Verification items for the finished model (mm, model axes). Face numbers are marked on the shaded views. A direction names the side the tool comes from. Give positions to 0.01 mm unless a question says otherwise; leave off trailing zeros. Write each loop counter-clockwise with the first axis right and the second up, starting at its lowest first coordinate (ties: lowest second). Pieces come first, ordered by that corner, then holes. Notation, with made-up numbers: (58, 9.25) - (108, 9.25) arc R15 cw to (108, 19.25) - close; hole circle Ø7 at (11, -34). An arc over 180 degrees is marked (long way). Put each result on its own line as item: value.
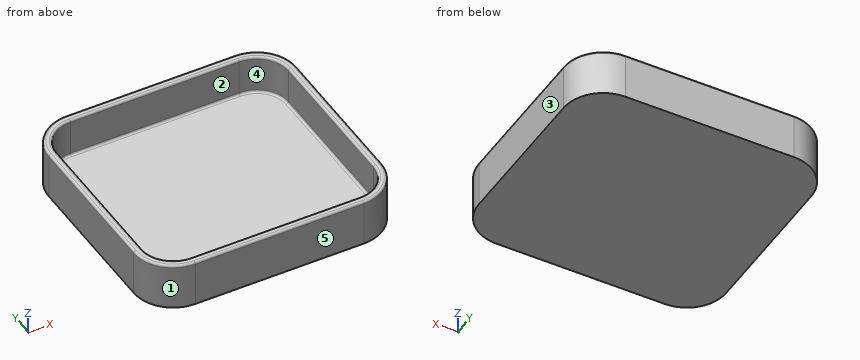
from build123d import *

# Parameters (mm, degrees)
F1_DEPTH = 2.5
F2_DEPTH = 15
F3_R     = 0.75


with BuildPart() as f1:
    # F0 (on Top) → F1 (new body)
    with BuildSketch(Plane.XY):
        with BuildLine():
            Line((26.75, 36.5), (-26.75, 36.5))
            ThreePointArc((-26.75, 36.5), (-35.5888347648, 32.8388347648), (-39.25, 24))
            Line((-39.25, 24), (-39.25, -24))
            ThreePointArc((-39.25, -24), (-35.5888347648, -32.8388347648), (-26.75, -36.5))
            Line((-26.75, -36.5), (26.75, -36.5))
            ThreePointArc((26.75, -36.5), (35.5888347648, -32.8388347648), (39.25, -24))
            Line((39.25, -24), (39.25, 24))
            ThreePointArc((39.25, 24), (35.5888347648, 32.8388347648), (26.75, 36.5))
        make_face()
        with BuildLine():
            ThreePointArc((-36.75, 24), (-33.8210678119, 31.0710678119), (-26.75, 34))
            Line((-26.75, 34), (26.75, 34))
            ThreePointArc((26.75, 34), (33.8210678119, 31.0710678119), (36.75, 24))
            Line((36.75, 24), (36.75, -24))
            ThreePointArc((36.75, -24), (33.8210678119, -31.0710678119), (26.75, -34))
            Line((26.75, -34), (-26.75, -34))
            ThreePointArc((-26.75, -34), (-33.8210678119, -31.0710678119), (-36.75, -24))
            Line((-36.75, -24), (-36.75, 24))
        make_face(mode=Mode.SUBTRACT)
        with BuildLine():
            Line((26.75, 34), (-26.75, 34))
            ThreePointArc((-26.75, 34), (-33.8210678119, 31.0710678119), (-36.75, 24))
            Line((-36.75, 24), (-36.75, -24))
            ThreePointArc((-36.75, -24), (-33.8210678119, -31.0710678119), (-26.75, -34))
            Line((-26.75, -34), (26.75, -34))
            ThreePointArc((26.75, -34), (33.8210678119, -31.0710678119), (36.75, -24))
            Line((36.75, -24), (36.75, 24))
            ThreePointArc((36.75, 24), (33.8210678119, 31.0710678119), (26.75, 34))
        make_face()
    extrude(amount=F1_DEPTH)

    # F0 (on Top) → F2 (join)
    with BuildSketch(Plane.XY):
        with BuildLine():
            Line((26.75, 36.5), (-26.75, 36.5))
            ThreePointArc((-26.75, 36.5), (-35.5888347648, 32.8388347648), (-39.25, 24))
            Line((-39.25, 24), (-39.25, -24))
            ThreePointArc((-39.25, -24), (-35.5888347648, -32.8388347648), (-26.75, -36.5))
            Line((-26.75, -36.5), (26.75, -36.5))
            ThreePointArc((26.75, -36.5), (35.5888347648, -32.8388347648), (39.25, -24))
            Line((39.25, -24), (39.25, 24))
            ThreePointArc((39.25, 24), (35.5888347648, 32.8388347648), (26.75, 36.5))
        make_face()
        with BuildLine():
            ThreePointArc((-36.75, 24), (-33.8210678119, 31.0710678119), (-26.75, 34))
            Line((-26.75, 34), (26.75, 34))
            ThreePointArc((26.75, 34), (33.8210678119, 31.0710678119), (36.75, 24))
            Line((36.75, 24), (36.75, -24))
            ThreePointArc((36.75, -24), (33.8210678119, -31.0710678119), (26.75, -34))
            Line((26.75, -34), (-26.75, -34))
            ThreePointArc((-26.75, -34), (-33.8210678119, -31.0710678119), (-36.75, -24))
            Line((-36.75, -24), (-36.75, 24))
        make_face(mode=Mode.SUBTRACT)
    extrude(amount=F2_DEPTH)

    # F3
    f3_edges = [f1.edges().sort_by_distance(p)[0] for p in [
        (0, 36.5, 15),
        (-35.588835, 32.838835, 15),
        (-39.25, 0, 15),
        (-35.588835, -32.838835, 15),
        (0, -36.5, 15),
        (35.588835, -32.838835, 15),
        (39.25, 0, 15),
        (35.588835, 32.838835, 15),
        (-33.821068, 31.071068, 15),
        (0, 34, 15),
        (33.821068, 31.071068, 15),
        (36.75, 0, 15),
        (33.821068, -31.071068, 15),
        (0, -34, 15),
        (-33.821068, -31.071068, 15),
        (-36.75, 0, 15),
        (-33.821068, 31.071068, 2.5),
        (0, 34, 2.5),
        (33.821068, 31.071068, 2.5),
        (36.75, 0, 2.5),
        (33.821068, -31.071068, 2.5),
        (0, -34, 2.5),
        (-33.821068, -31.071068, 2.5),
        (-36.75, 0, 2.5),
    ]]
    fillet(f3_edges, radius=F3_R)


solid = f1.part
Q1. Section check C-C, the plane x = -12. Record the cut outline in (y, z), plus the area to 3 significant figures.
Answers follow:
outline: (-36.5, 0) - (36.5, 0) - (36.5, 14.25) arc R0.75 ccw to (35.75, 15) - (34.75, 15) arc R0.75 ccw to (34, 14.25) - (34, 3.25) arc R0.75 cw to (33.25, 2.5) - (-33.25, 2.5) arc R0.75 cw to (-34, 3.25) - (-34, 14.25) arc R0.75 ccw to (-34.75, 15) - (-35.75, 15) arc R0.75 ccw to (-36.5, 14.25) - close
area: 245 mm2
Q2. Release check for a two-part mould opening along Y. For the marked faces 3, 4 and 5 record: released by +Y, released by -Y, zero draft, split by the parting line, or undercut.
Answers follow:
face 3: zero draft
face 4: undercut
face 5: released by -Y
Q3. Go/stop test with a flat-tipped pin: pin 1 Ø10 at (x, y) = (-8.5, -22.5) entering from +Z. Record where the tip stops, or that it passes through.
Answers follow:
pin 1: stops at z = 2.5
Q4. Set-up check for the marked faces 1 and 2: record each of +Z, -Z, +X, -X, +Y, -Y from which the full face is reachable in a straight line by a thin tool's end or side.
Answers follow:
face 1: +Z, -Z, -X, -Y
face 2: +Z
Q5. Section check B-B, the plane y = -20. Record the cut outline in (x, z).
Answers follow:
outline: (-39.25, 0) - (39.25, 0) - (39.25, 14.25) arc R0.75 ccw to (38.5, 15) - (37.5, 15) arc R0.75 ccw to (36.75, 14.25) - (36.75, 3.25) arc R0.75 cw to (36, 2.5) - (-36, 2.5) arc R0.75 cw to (-36.75, 3.25) - (-36.75, 14.25) arc R0.75 ccw to (-37.5, 15) - (-38.5, 15) arc R0.75 ccw to (-39.25, 14.25) - close
Q6. Section check A-A, the plane z = 10. Record the cut outline in (x, y).
Answers follow:
outline: (-39.25, -24) arc R12.5 ccw to (-26.75, -36.5) - (26.75, -36.5) arc R12.5 ccw to (39.25, -24) - (39.25, 24) arc R12.5 ccw to (26.75, 36.5) - (-26.75, 36.5) arc R12.5 ccw to (-39.25, 24) - close; hole (-36.75, -24) arc R10 ccw to (-26.75, -34) - (26.75, -34) arc R10 ccw to (36.75, -24) - (36.75, 24) arc R10 ccw to (26.75, 34) - (-26.75, 34) arc R10 ccw to (-36.75, 24) - close
Q7. Scan lines: line 1 along Y through (x, z) = (18, 5.25); line 2 along X through (y, z) = (-21.5, 6.75); line 3 along Z through (x, y) = (-8, 23). Record each from-to range of solid material in increasing order.
Answers follow:
line 1: y = -36.5 to -34, 34 to 36.5
line 2: x = -39.25 to -36.75, 36.75 to 39.25
line 3: z = 0 to 2.5
